from build123d import *

# Parameters (mm, degrees)
SKETCH_1_W          = 5.8
SKETCH_1_H          = 5.8
EXTRUDE_1_DEPTH     = 2.2
SKETCH_3_W          = 3.7
SKETCH_3_H          = 3
CUT_EXTRUDE_2_DEPTH = 1.75
CUT_EXTRUDE_START   = -0.8
CUT_EXTRUDE_1_DEPTH = 4.854030511
CHAMFER_1_SIZE      = 0.24


with BuildPart() as part:
    # 草图1 → 凸台-拉伸1 (new body)
    with BuildSketch(Plane(origin=(0, 0, 0), x_dir=(1, 0, 0), z_dir=(0, 1, 0))):
        Rectangle(SKETCH_1_W, SKETCH_1_H)
    extrude(amount=EXTRUDE_1_DEPTH)

    # 草图3 → 切除-拉伸2 (cut)
    with BuildSketch(Plane.XZ):
        Rectangle(SKETCH_3_W, SKETCH_3_H)
    extrude(amount=-CUT_EXTRUDE_2_DEPTH, mode=Mode.SUBTRACT)

    # 草图2 → 切除-拉伸1 (cut, through all)
    with BuildSketch(Plane.XZ.offset(CUT_EXTRUDE_START)):
        Polygon((-2.9, 2.3), (-2.9, -2.3), (-2.5, -1.9), (-2.5, 1.9), align=None)
        Polygon((-1.9, 2.5), (-2.3, 2.9), (2.3, 2.9), (1.9, 2.5), align=None)
        Polygon((2.5, 1.9), (2.9, 2.3), (2.9, -2.3), (2.5, -1.9), align=None)
        Polygon((1.9, -2.5), (2.3, -2.9), (-2.3, -2.9), (-1.9, -2.5), align=None)
    extrude(amount=-CUT_EXTRUDE_1_DEPTH, mode=Mode.SUBTRACT)

    # 倒角1
    chamfer_1_edges = [part.edges().sort_by_distance(p)[0] for p in [
        (-2.5, 2.2, 0),
        (0, 2.2, 2.5),
        (2.5, 2.2, 0),
        (0, 2.2, -2.5),
    ]]
    chamfer(chamfer_1_edges, length=CHAMFER_1_SIZE)


solid = part.part
Read the model definition and answer for the solid it produces. Units are mm, in the model's axes. A direction names the side the tool comes from. Give positions to 0.01 mm unless a question says otherwise; leave off trailing zeros. Write each loop counter-clockwise with the first axis right and the second up, starting at its lowest first coordinate (ties: lowest second). Pieces come first, ordered by that corner, then holes. Notation, with made-up numbers: M 60,76 L 116,76 A7 cw 116,86 Z; hole C 88,53 d5. An arc over 180 degrees is marked long. One line per item, written item: value. Start each with the question number.
(1) Find the intervals of material crossed by line 1 (Z direction, x = 1.55, y = 0.7); line 2 (X direction, y = 0.3, z = -0.9); line 3 (Z direction, x = 1.35, y = 1.05), in increasing order.
(2) Find section A-A (y = 0.5). Determine the outline of the cut face in (x, z).
(3) A tool of negligible diameter and unlimited length cuts with its end or side. For faces 1 (the flat face through (2.9, 0.6, 0)), 2 (the flat face through (0, 1, -2.5)), 3 (the flat face through (2.5, 1, 0)), 4 (the flat face through (0, 1.75, 0)), from which of +Z, -Z, +X, -X, +Y, -Y can it reach the whole face along a straight path? Write none if from no direction.
(4) Find section C-C (x = 1.5). Determine the outline of the cut face in (y, z), plus the area to 3 significant figures.
(5) Find section D-D (y = 1.05). Determine the outline of the cut face in (x, z), plus the area to 3 significant figures.
(6) Determine the mould class of faces 5 (the flat face through (0, 0.6, -2.9)), 6 (the flat face through (0, 1, 2.5)), 7 (the flat face through (-2.5, 1, 0)) for opening direction X: pulls with the +X half, pulls with the -X half, needs draft (parallel to the pull), parting line crosses it, or undercut.
(7) Find section B-B (z = 2.15). Determine the outline of the cut face in (x, y), plus the area to 3 significant figures.
(8) Flat-ended cylindrical pins translate along their axes: pin 1 Ø1.3 at (y, z) = (1, -1) entering from -X; pin 2 Ø2.5 at (x, z) = (0, 0) entering from -Y. Find the tip coordinate at first contact, or state that the pin passes through.
Results below:
1. line 1: z = -2.9 to -1.5, 1.5 to 2.9
1. line 2: x = -2.9 to -1.85, 1.85 to 2.9
1. line 3: z = -2.5 to -1.5, 1.5 to 2.5
2. outline: M -2.9,-2.9 L 2.9,-2.9 L 2.9,2.9 L -2.9,2.9 Z; hole M -1.85,-1.5 L 1.85,-1.5 L 1.85,1.5 L -1.85,1.5 Z
3. face 1: +Z, -Z, +X, +Y, -Y
3. face 2: -Z, +Y
3. face 3: +X, +Y
3. face 4: -Y
4. outline: M 0,-2.9 L 0.8,-2.9 L 0.8,-2.5 L 1.96,-2.5 L 2.2,-2.26 L 2.2,2.26 L 1.96,2.5 L 0.8,2.5 L 0.8,2.9 L 0,2.9 L 0,1.5 L 1.75,1.5 L 1.75,-1.5 L 0,-1.5 Z
4. area: 6.33 mm^2
5. outline: M -2.9,-2.9 L -2.3,-2.9 L -1.9,-2.5 L 1.9,-2.5 L 2.3,-2.9 L 2.9,-2.9 L 2.9,-2.3 L 2.5,-1.9 L 2.5,1.9 L 2.9,2.3 L 2.9,2.9 L 2.3,2.9 L 1.9,2.5 L -1.9,2.5 L -2.3,2.9 L -2.9,2.9 L -2.9,2.3 L -2.5,1.9 L -2.5,-1.9 L -2.9,-2.3 Z; hole M -1.85,-1.5 L 1.85,-1.5 L 1.85,1.5 L -1.85,1.5 Z
5. area: 15.8 mm^2
6. face 5: needs draft
6. face 6: undercut
6. face 7: pulls with the -X half
7. outline: M -2.9,0 L 2.9,0 L 2.9,0.8 L 2.75,0.8 L 2.75,2.2 L -2.75,2.2 L -2.75,0.8 L -2.9,0.8 Z
7. area: 12.3 mm^2
8. pin 1: stops at x = -2.9
8. pin 2: stops at y = 1.75
